Design review of the part built by this model. Coordinates are the model's own, in mm. Give positions to 0.01 mm unless a question says otherwise; leave off trailing zeros. Loops run counter-clockwise (first coordinate to the right, second up) from the corner with the lowest first, then second, coordinate; pieces in that order, holes last. Notation, with made-up numbers: (17, 34) -> (26, 34) arc R29 cw to (26, 64) -> close; hole circle Ø8 at (35, 66.25). An arc over 180 degrees is marked (long way). Use a Markdown table: item, result. Add a question column.
1. Add section A-A (z = 2.2). State the section outline as (x, y) points, and give its area (3 significant figures).
2. Draft analysis for pull direction X (two halves, no side actions). For faces 1 (the cylindrical face through (-87.001, -290.243, 1.972)), 2 (the flat face through (-14, -322, 0)), 3 (the cylindrical face through (105.535, -381.822, 1.972)), 4 (the cylindrical face through (-136.06, -263.44, 1.97)), state which applies: pulls with the +X half, pulls with the -X half, needs draft (parallel to the pull), parting line crosses it, or undercut.
3. To check wall thickness, follow line 1 (Y direction, x = -87.5, z = 1.6); line 2 (X direction, y = -345, z = 1.5); line 3 (X direction, y = -346, z = 0.35). State the ranges of each line that lie inside material, in increasing order.
```python
from build123d import *

# Parameters (mm, degrees)
BOSS_EXTRUDE1_DEPTH  = 4
M6_CLEARANCE_HOLE1_D = 6.4
SKETCH5_R            = 7.5
CUT_EXTRUDE1_DEPTH   = 40.678061403


with BuildPart() as part:
    # Sketch1 → Boss-Extrude1 (new body)
    with BuildSketch(Plane.XY):
        with BuildLine():
            Line((98.386811049, -384.8287802), (-128.910956341, -384.8287802))
            ThreePointArc((-128.910956341, -384.8287802), (-135.982024153, -381.899848012), (-138.910956341, -374.8287802))
            Line((-138.910956341, -374.8287802), (-138.910956341, -270.434125192))
            ThreePointArc((-138.910956341, -270.434125192), (-135.982024153, -263.36305738), (-128.910956341, -260.434125192))
            Line((-128.910956341, -260.434125192), (98.386811049, -260.434125192))
            ThreePointArc((98.386811049, -260.434125192), (105.457878861, -263.36305738), (108.386811049, -270.434125192))
            Line((108.386811049, -270.434125192), (108.386811049, -374.8287802))
            ThreePointArc((108.386811049, -374.8287802), (105.457878861, -381.899848012), (98.386811049, -384.8287802))
        make_face()
    extrude(amount=BOSS_EXTRUDE1_DEPTH)

    # M6 Clearance Hole1 (through all)
    with Locations(Plane.XY.offset(4)):
        with Locations((54.16270611, -293.415681156), (54.16270611, -321.915681156), (45.426427008, -344.165502047), (-78.681014788, -344.165502047), (-87.41729389, -321.915681156), (-87.41729389, -293.415681156)):
            Hole(M6_CLEARANCE_HOLE1_D / 2)

    # Sketch5 → Cut-Extrude1 (cut)
    with BuildSketch(Plane.XY.offset(4)):
        with Locations((-78.681014788, -344.165502047)):
            Circle(SKETCH5_R)
        with Locations((45.426427008, -344.165502047)):
            Circle(SKETCH5_R)
    extrude(amount=-CUT_EXTRUDE1_DEPTH, mode=Mode.SUBTRACT)


solid = part.part
```
Taken from the geometry:
| question | item | result |
|---|---|---|
| 1 | outline | (-138.91, -374.83) arc R10 ccw to (-128.91, -384.83) -> (98.39, -384.83) arc R10 ccw to (108.39, -374.83) -> (108.39, -270.43) arc R10 ccw to (98.39, -260.43) -> (-128.91, -260.43) arc R10 ccw to (-138.91, -270.43) -> close; hole circle Ø6.4 at (-87.42, -321.92); hole circle Ø6.4 at (-87.42, -293.42); hole circle Ø15 at (-78.68, -344.17); hole circle Ø15 at (45.43, -344.17); hole circle Ø6.4 at (54.16, -321.92); hole circle Ø6.4 at (54.16, -293.42) |
| 1 | area | 30,200 mm^2 |
| 2 | face 1 | undercut |
| 2 | face 2 | needs draft |
| 2 | face 3 | pulls with the +X half |
| 2 | face 4 | pulls with the -X half |
| 3 | line 1 | y = -384.83 to -325.11, -318.72 to -296.61, -290.22 to -260.43 |
| 3 | line 2 | x = -138.91 to -86.13, -71.23 to 37.97, 52.88 to 108.39 |
| 3 | line 3 | x = -138.91 to -85.95, -71.41 to 38.15, 52.7 to 108.39 |
